The listing builds one solid part. Answer for the finished solid, in the listing's coordinates (mm). A direction names the side the tool comes from. Round coordinates to 2 decimals unless told otherwise and drop trailing zeros. Write each loop counter-clockwise with the first axis right and the second up, starting at its lowest first coordinate (ties: lowest second). Pieces come first, ordered by that corner, then holes. Notation, with made-up numbers: (1, -11.75) - (13, -11.75) arc R27 ccw to (13, 12.25) - close; hole circle Ø8 at (0.5, 76). An arc over 180 degrees is marked (long way). Answer in a Markdown table with one row per item.
from build123d import *

# Parameters (mm, degrees)
SKETCH1_R                                         = 1.4732
BOSS_EXTRUDE1_DEPTH                               = 3.175
BOSS_EXTRUDE2_START                               = 2.54
BOSS_EXTRUDE2_DEPTH                               = 2.54
CSK_FOR_4_FLAT_HEAD_MACHINE_SCREW_100_D           = 2.9464
CSK_FOR_4_FLAT_HEAD_MACHINE_SCREW_100_CSINK_D     = 7.2285352
CSK_FOR_4_FLAT_HEAD_MACHINE_SCREW_100_CSINK_ANGLE = 100


with BuildPart() as part:
    # Sketch1 → Boss-Extrude1 (new body)
    with BuildSketch(Plane(origin=(0, 0, 0), x_dir=(1, 0, 0), z_dir=(0, 1, 0))):
        with BuildLine():
            Line((-10.119178406, -0.909850746), (-6.324486504, -43.113656716))
            ThreePointArc((-6.324486504, -43.113656716), (0, -48.895), (6.324486504, -43.113656716))
            Line((6.324486504, -43.113656716), (10.119178406, -0.909850746))
            ThreePointArc((10.119178406, -0.909850746), (0, 10.16), (-10.119178406, -0.909850746))
        make_face()
        with Locations(Location((0, -42.545, 0), (0, 0, 270))):
            Circle(SKETCH1_R, mode=Mode.SUBTRACT)
    extrude(amount=BOSS_EXTRUDE1_DEPTH)

    # Sketch2 → Boss-Extrude2 (add)
    with BuildSketch(Plane.XZ.offset(BOSS_EXTRUDE2_START)):
        with BuildLine():
            Line((7.62, 0), (10.16, 0))
            ThreePointArc((10.16, 0), (0, 10.16), (-10.16, 0))
            Line((-10.16, 0), (-7.62, 0))
            ThreePointArc((-7.62, 0), (0, -7.62), (7.62, 0))
        make_face()
    extrude(amount=-BOSS_EXTRUDE2_DEPTH)

    # CSK for #4 Flat Head Machine Screw (100)1 (through all)
    with Locations(Plane(origin=(0, 3.175, 0), x_dir=(1, 0, 0), z_dir=(0, 1, 0))):
        with Locations((0, 0)):
            CounterSinkHole(CSK_FOR_4_FLAT_HEAD_MACHINE_SCREW_100_D / 2, CSK_FOR_4_FLAT_HEAD_MACHINE_SCREW_100_CSINK_D / 2, counter_sink_angle=CSK_FOR_4_FLAT_HEAD_MACHINE_SCREW_100_CSINK_ANGLE)


solid = part.part
(1) Section A-A (x = 0) is taken. Give the vertices of the cut face in (y, z) (3 decimals), and give its area (3 significant figures).
Checked values:
| item | result |
|---|---|
| outline | (-2.54, -7.62) - (0, -7.62) - (0, -10.16) - (3.175, -10.16) - (3.175, -3.614) - (1.378, -1.473) - (-2.54, -1.473) - close; (-2.54, 1.473) - (1.378, 1.473) - (3.175, 3.614) - (3.175, 41.072) - (0, 41.072) - (0, 10.16) - (-2.54, 10.16) - close; (0, 44.018) - (3.175, 44.018) - (3.175, 48.895) - (0, 48.895) - close |
| area | 203 mm2 |
(2) Section D-D (x = 5.25) is taken. Give the vertices of the cut face in (y, z) (3 decimals).
Checked values:
| item | result |
|---|---|
| outline | (-2.54, -5.523) - (0, -5.523) - (0, -8.698) - (3.175, -8.698) - (3.175, 46.117) - (0, 46.117) - (0, 8.698) - (-2.54, 8.698) - close |
(3) Section B-B (y = -1.1) is taken. Give the vertices of the cut face in (x, z).
Checked values:
| item | result |
|---|---|
| outline | (-10.16, 0) - (-7.62, 0) arc R7.62 ccw to (7.62, 0) - (10.16, 0) arc R10.16 ccw to start; hole circle Ø2.95 at (0, 0) |
(4) Section C-C (z = -5.5) is taken. Give the vertices of the cut face in (x, y) (3 decimals).
Checked values:
| item | result |
|---|---|
| outline | (-8.543, 0) - (-5.274, 0) - (-5.274, -2.54) - (5.274, -2.54) - (5.274, 0) - (8.543, 0) - (8.543, 3.175) - (-8.543, 3.175) - close |
(5) Find the intervals of material crossed by line 1 (Y direction, x = -1.5, z = 28) (3 decimals); line 2 (X direction, y = 1.8, z = -1); line 3 (Y direction, x = 3, z = 2), in increasing order.
Checked values:
| item | result |
|---|---|
| line 1 | y = 0 to 3.175 |
| line 2 | x = -10.11 to -1.7, 1.7 to 10.11 |
| line 3 | y = -2.54 to 3.17 |
(6) For faces 1 (the flat face through (0, 0, -9)), 2 (the flat face through (9, -1, 0)), 3 (the flat face through (-9, -1, 0)), determine the directions among +Z, -Z, +X, -X, +Y, -Y from which every point of the face is accessible in a straight line to the end or side of a thin tool.
Checked values:
| item | result |
|---|---|
| face 1 | -Z, -Y |
| face 2 | -Z, +X, -Y |
| face 3 | -Z, -X, -Y |
(7) For a pull along X with two mould halves and no side action, classify faces 4 (the conical face through (-1.5, 1.5, 0.6)), 5 (the flat face through (0, 0, 25)), 6 (the cylindrical face through (-0.17, -1.29, -7.62)) as pulls with the +X half, pulls with the -X half, needs draft (parallel to the pull), parting line crosses it, or undercut.
Checked values:
| item | result |
|---|---|
| face 4 | undercut |
| face 5 | needs draft |
| face 6 | parting line crosses it |
(8) Flat-ended cylindrical pins translate along their axes: pin 1 (0.8 mm diameter, centred on x = -9, y = -1, fed in from -Z); pin 2 (3.5 mm diameter, centred on x = 0, z = 0, fed in from -Y). Find the tip coordinate at first contact, or state that the pin passes through.
Checked values:
| item | result |
|---|---|
| pin 1 | stops at z = 0 |
| pin 2 | stops at y = -2.54 |
